Here's how the part is built. I have some questions about the finished solid (model axes, mm). Face numbers are marked on the shaded views. A direction names the side the tool comes from. Coordinates: 2 decimals unless noted, no trailing zeros. Loops run counter-clockwise (first coordinate to the right, second up) from the corner with the lowest first, then second, coordinate; pieces in that order, holes last.
from build123d import *

# Parameters (mm, degrees)
SKETCH1_R               = 6
BOSS_EXTRUDE1_DEPTH     = 2
SKETCH2_R               = 4
BOSS_EXTRUDE2_DEPTH     = 2
SKETCH3_R               = 2.1
CUT_EXTRUDE1_DEPTH      = 1
CUT_EXTRUDE1_DEPTH_BACK = 5
SKETCH4_R               = 3.5
SKETCH4_R_2             = 2.1
BOSS_EXTRUDE3_DEPTH     = 1


with BuildPart() as part:
    # Sketch1 → Boss-Extrude1 (new body)
    with BuildSketch(Plane(origin=(0, 0, 0), x_dir=(1, 0, 0), z_dir=(0, 1, 0))):
        Circle(SKETCH1_R)
    extrude(amount=BOSS_EXTRUDE1_DEPTH)

    # Sketch2 → Boss-Extrude2 (add)
    with BuildSketch(Plane(origin=(0, 2, 0), x_dir=(1, 0, 0), z_dir=(0, 1, 0))):
        Circle(SKETCH2_R)
    extrude(amount=BOSS_EXTRUDE2_DEPTH)

    # Sketch3 → Cut-Extrude1 (cut, two sides)
    with BuildSketch(Plane(origin=(0, 4, 0), x_dir=(1, 0, 0), z_dir=(0, 1, 0))) as cut_extrude1_sk:
        Circle(SKETCH3_R)
    extrude(amount=CUT_EXTRUDE1_DEPTH, mode=Mode.SUBTRACT)
    extrude(cut_extrude1_sk.sketch, amount=-CUT_EXTRUDE1_DEPTH_BACK, mode=Mode.SUBTRACT)

    # Sketch4 → Boss-Extrude3 (add)
    with BuildSketch(Plane.XZ):
        Circle(SKETCH4_R)
        Circle(SKETCH4_R_2, mode=Mode.SUBTRACT)
    extrude(amount=BOSS_EXTRUDE3_DEPTH)


solid = part.part
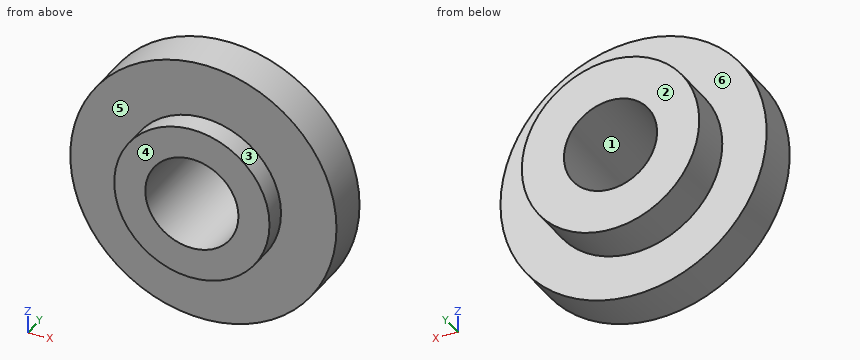
Q1. Suppose I cut it at B-B on x = 0. Write out the boundary of the cut face in (y, z), and give its area (3 significant figures).
Q2. We'd pull the mould along X, two halves only. Please class the marked faces 1, 2 and 3: pulls with the +X half, pulls with the -X half, needs draft (parallel to the pull), parting line crosses it, or undercut.
Q3. Please list where these lines run through material, in increasing order: probe 1 along X at (y, z) = (1.85, 0); probe 2 along Z at (x, y) = (0, 2.6).
Q4. Will these pins go through, and if not, where does the flat tip stop? P1, Ø3, axis at x = 3, y = 3, coming from the +Z side; P2, Ø1, axis at y = 3.5, z = 2.5, coming from the +X side.
Q5. Suppose I cut it at D-D on z = -3.75. Write out the boundary of the cut face in (x, y).
Q6. Suppose I cut it at C-C on y = 1.5. Write out the boundary of the cut face in (x, z).
Q7. Suppose I cut it at A-A on z = 0. Write out the boundary of the cut face in (x, y).
Q8. For the marked faces 4, 5 and 6, which set-ups out of +Z, -Z, +X, -X, +Y, -Y let a thin tool reach every point of the face, with its end or its side?
Check values:
1. outline: (-1, -3.5) - (0, -3.5) - (0, -6) - (2, -6) - (2, -4) - (4, -4) - (4, -2.1) - (-1, -2.1) - close; (-1, 2.1) - (4, 2.1) - (4, 4) - (2, 4) - (2, 6) - (0, 6) - (0, 3.5) - (-1, 3.5) - close
1. area: 26.0 mm2
2. face 1: undercut
2. face 2: needs draft
2. face 3: parting line crosses it
3. probe 1: x = -6 to -2.1, 2.1 to 6
3. probe 2: z = -4 to -2.1, 2.1 to 4
4. P1: stops at z = 5.7
4. P2: stops at x = 3.46
5. outline: (-4.68, 0) - (4.68, 0) - (4.68, 2) - (1.39, 2) - (1.39, 4) - (-1.39, 4) - (-1.39, 2) - (-4.68, 2) - close
6. outline: circle Ø12 at (0, 0); hole circle Ø4.2 at (0, 0)
7. outline: (-6, 0) - (-3.5, 0) - (-3.5, -1) - (-2.1, -1) - (-2.1, 4) - (-4, 4) - (-4, 2) - (-6, 2) - close; (2.1, -1) - (3.5, -1) - (3.5, 0) - (6, 0) - (6, 2) - (4, 2) - (4, 4) - (2.1, 4) - close
8. face 4: +Z, -Z, +X, -X, -Y
8. face 5: -Y
8. face 6: +Y
